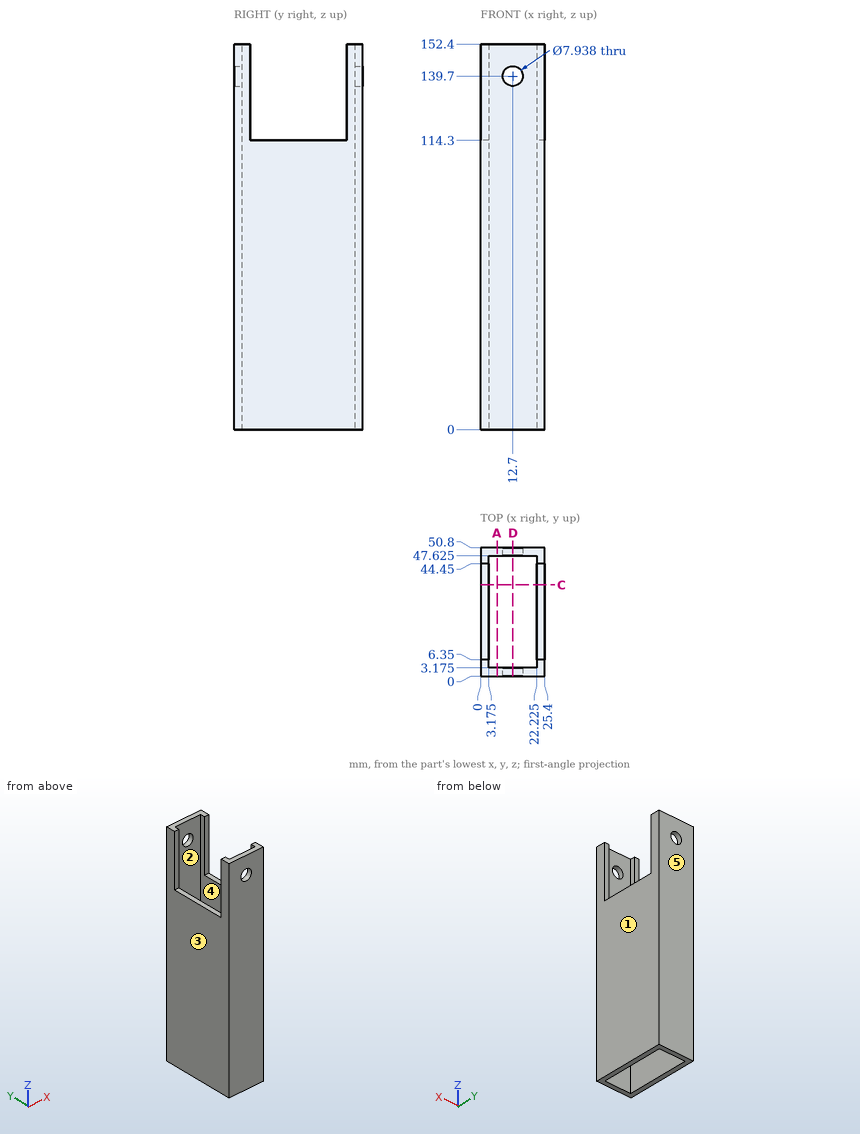
Print and shaded views of the part. All mm, measured from the part's lowest x, y and z. A direction names the side the tool comes from. Round coordinates to 2 decimals unless told otherwise and drop trailing zeros. Write each loop counter-clockwise with the first axis right and the second up, starting at its lowest first coordinate (ties: lowest second). Pieces come first, ordered by that corner, then holes. Notation, with made-up numbers: (46.25, 6.25) - (94.25, 6.25) arc R20 ccw to (94.25, 13.25) - close; hole circle Ø11 at (59, 7.5). An arc over 180 degrees is marked (long way). One line per item, written item: value.
(1) Cut at D-D, the plane x = 12.7. Give the cut face in (y, z) (1 decimal).
Values follow:
outline: (0, 0) - (3.2, 0) - (3.2, 135.7) - (0, 135.7) - close; (0, 143.7) - (3.2, 143.7) - (3.2, 152.4) - (0, 152.4) - close; (47.6, 0) - (50.8, 0) - (50.8, 135.7) - (47.6, 135.7) - close; (47.6, 143.7) - (50.8, 143.7) - (50.8, 152.4) - (47.6, 152.4) - close
(2) Drop a flat-ended pin along its axis: P1, Ø3.5, axis at x = 24.5, y = 19.5, coming from the +Z side. Give the stop position or say it passes through.
Values follow:
P1: stops at z = 114.3
(3) Cut at A-A, the plane x = 6.5. Give the cut face in (y, z) (1 decimal).
Values follow:
outline: (0, 0) - (3.2, 0) - (3.2, 152.4) - (0, 152.4) - close; (47.6, 0) - (50.8, 0) - (50.8, 152.4) - (47.6, 152.4) - close
(4) Wall check: probe 1 along Z at (x, y) = (12.7, 1); probe 2 along Y at (x, z) = (9.75, 33) (1 decimal); probe 3 along X at (y, z) = (21, 44) (1 decimal). Give the ranges that are in metal, low to high.
Values follow:
probe 1: z = 0 to 135.73, 143.67 to 152.4
probe 2: y = 0 to 3.2, 47.6 to 50.8
probe 3: x = 0 to 3.2, 22.2 to 25.4
(5) Two-plate mould, pull along Y, no slides. Class the marked faces 3, 4 and 5: pulls with the +Y half, pulls with the -Y half, needs draft (parallel to the pull), parting line crosses it, or undercut.
Values follow:
face 3: needs draft
face 4: undercut
face 5: pulls with the +Y half
(6) 3-axis set-ups, long thin cutter, end or side, ignore diameter. For the marked faces 1 and 2: which of +Z, -Z, +X, -X, +Y, -Y reach the whole face in a straight line?
Values follow:
face 1: +Z, -Z, +X, +Y, -Y
face 2: +Z, -Z
(7) Cut at C-C, the plane y = 36. Give the cut face in (x, z) (1 decimal).
Values follow:
outline: (0, 0) - (3.2, 0) - (3.2, 114.3) - (0, 114.3) - close; (22.2, 0) - (25.4, 0) - (25.4, 114.3) - (22.2, 114.3) - close
